CAD build for the part. Positions are in the model's coordinates, mm. Coordinates: 2 decimals unless noted, no trailing zeros. Loops run counter-clockwise (first coordinate to the right, second up) from the corner with the lowest first, then second, coordinate; pieces in that order, holes last. Notation, with made-up numbers: (79.25, 45.25) -> (135.25, 45.25) arc R10 ccw to (135.25, 53.25) -> close; hole circle Ø4 at (86, 20). An arc over 180 degrees is marked (long way). Write each question's results on one line, items separated by ' | '.
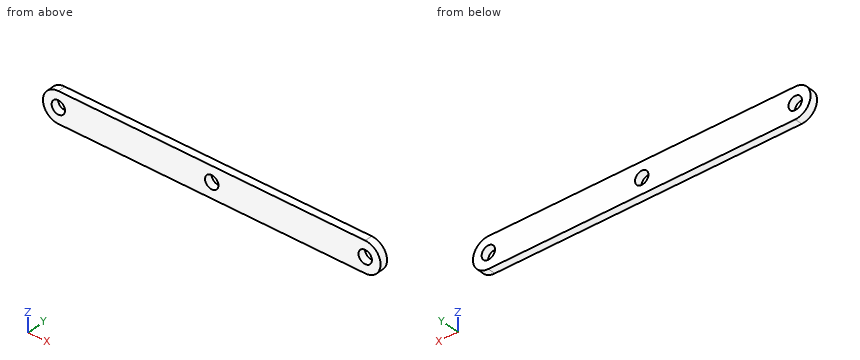
```python
from build123d import *

# Parameters (mm, degrees)
EXTRUDE_1_DEPTH     = 2
SKETCH_2_R          = 1.75
CUT_EXTRUDE_1_DEPTH = 50.107311212


with BuildPart() as part:
    # 草图1 → 凸台-拉伸1 (new body)
    with BuildSketch(Plane(origin=(0, 0, 0), x_dir=(1, 0, 0), z_dir=(0, 1, 0))):
        with BuildLine():
            Line((-44.903251574, 4), (35.096748426, 4))
            ThreePointArc((35.096748426, 4), (39.096748426, 0), (35.096748426, -4))
            Line((35.096748426, -4), (-44.903251574, -4))
            ThreePointArc((-44.903251574, -4), (-48.903251574, 0), (-44.903251574, 4))
        make_face()
    extrude(amount=EXTRUDE_1_DEPTH)

    # 草图2 → 切除-拉伸1 (cut, through all)
    with BuildSketch(Plane(origin=(0, 2, 0), x_dir=(1, 0, 0), z_dir=(0, 1, 0))):
        with Locations(Location((-44.903251574, 0, 0), (0, 0, 270))):
            Circle(SKETCH_2_R)
        with Locations(Location((35.096748426, 0, 0), (0, 0, 270))):
            Circle(SKETCH_2_R)
        with Locations(Location((-4.903251574, 0, 0), (0, 0, 270))):
            Circle(SKETCH_2_R)
    extrude(amount=-CUT_EXTRUDE_1_DEPTH, mode=Mode.SUBTRACT)


solid = part.part
```
Q1. Drop a flat-ended pin along its axis: pin 1 (2 mm diameter, centred on x = 35.1, z = 0, fed in from +Y). Give the stop position or say it passes through.
Results are:
pin 1: through
Q2. Cut at A-A on z = 0. Write the cut outline in (x, y), and give its area (3 significant figures).
Results are:
outline: (-48.9, 0) -> (-46.65, 0) -> (-46.65, 2) -> (-48.9, 2) -> close; (-43.15, 0) -> (-6.65, 0) -> (-6.65, 2) -> (-43.15, 2) -> close; (-3.15, 0) -> (33.35, 0) -> (33.35, 2) -> (-3.15, 2) -> close; (36.85, 0) -> (39.1, 0) -> (39.1, 2) -> (36.85, 2) -> close | area: 155 mm^2
Q3. Wall check: L1, parallel to X at y = 1.35, z = 0; L2, parallel to X at y = 1, z = 0.5; L3, parallel to X at y = 0.15, z = 2.75. Give the ranges that are in metal, low to high. Write a range as from..to.
Results are:
L1: -48.9..-46.65, -43.15..-6.65, -3.15..33.35, 36.85..39.1 | L2: -48.87..-46.58, -43.23..-6.58, -3.23..33.42, 36.77..39.07 | L3: -47.81..38
Q4. Cut at B-B on z = -3.25. Write the cut outline in (x, y).
Results are:
outline: (-47.24, 0) -> (37.43, 0) -> (37.43, 2) -> (-47.24, 2) -> close
